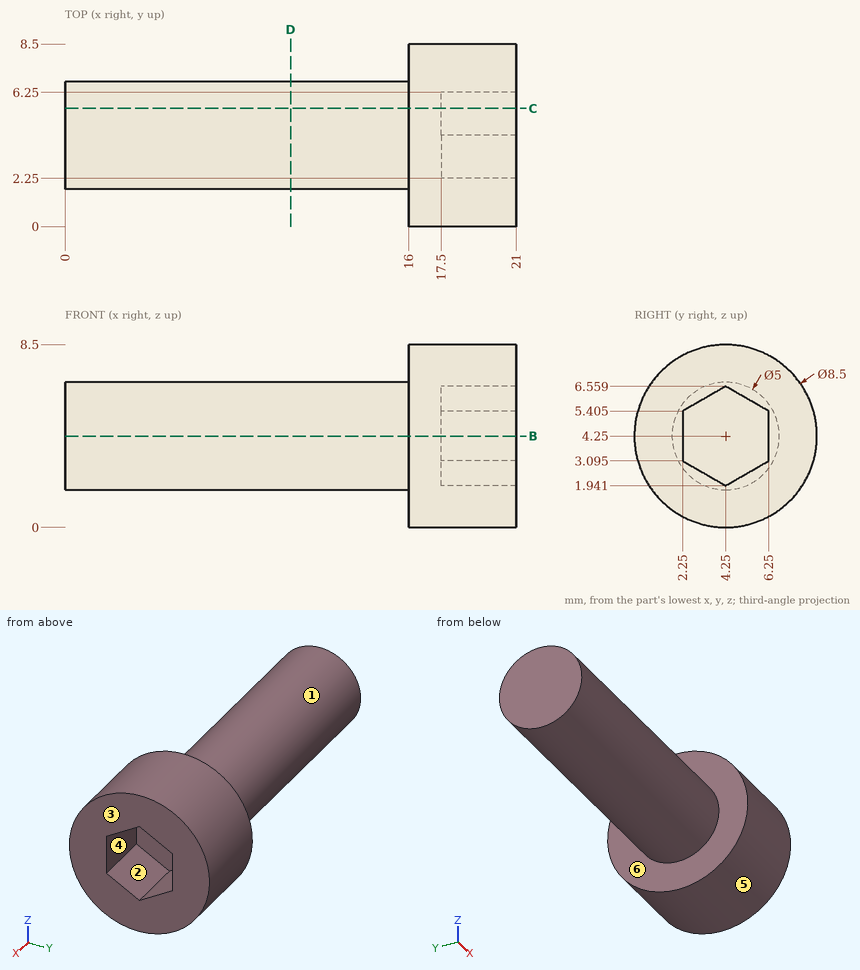
Study the drawing (mm; zero at the part's minimum x, y, z) and answer. A direction names the side the tool comes from. Give positions to 0.01 mm unless a question says otherwise; leave off trailing zeros. Write each loop counter-clockwise with the first axis right and the second up, starting at its lowest first coordinate (ties: lowest second). Pieces come first, ordered by that corner, then holes. Notation, with made-up numbers: (56.25, 73) - (78.25, 73) arc R30 cw to (78.25, 108) - close; hole circle Ø11 at (-4.75, -17). An arc over 180 degrees is marked (long way). Use CSV: the item, a comma, the result in double quotes. Start each with the question number.
(1) Find section C-C (y = 5.5). Give the vertices of the cut face in (x, z) (1 decimal).
(2) Find section D-D (x = 10.5). Give the vertices of the cut face in (y, z).
(3) Given P1, Ø2, axis at x = 11.5, y = 6.5, coming from the -Z side (1 decimal); P2, Ø1, axis at x = 11.5, y = 2, coming from the -Z side (1 decimal); P3, Ø1, axis at x = 7, z = 2.5, coming from the +Y side (1 decimal), each flat-ended and moving along its own axis, determine where each tip first touches the part or whether it passes through.
(4) Determine the mould class of the marked faces 4, 5 and 6 for opening direction Z: +Z half, -Z half, draft (parallel to the pull), parting line (faces both ways), or undercut.
(5) For the marked faces 1, 2 and 3, determine the directions among +Z, -Z, +X, -X, +Y, -Y from which every point of the face is accessible in a straight line to the end or side of a thin tool.
(6) Consider line 1 along X through (y, z) = (3, 1.75); line 2 along Z through (x, y) = (19, 0.5); line 3 along Y through (x, z) = (19.25, 1.25). Determine where each line is inside the solid, lowest interval first.
(7) Find section B-B (z = 4.25). Give the vertices of the cut face in (x, y).
Findings below:
1,outline,"(0, 2.1) - (16, 2.1) - (16, 0.2) - (21, 0.2) - (21, 2.7) - (17.5, 2.7) - (17.5, 5.8) - (21, 5.8) - (21, 8.3) - (16, 8.3) - (16, 6.4) - (0, 6.4) - close"
2,outline,"circle Ø5 at (4.25, 4.25)"
3,P1,"z = 2.1"
3,P2,"z = 2.5"
3,P3,"y = 6.4"
4,face 4,"undercut"
4,face 5,"parting line"
4,face 6,"draft"
5,face 1,"-X"
5,face 2,"+X"
5,face 3,"+Z, -Z, +X, +Y, -Y"
6,line 1,"16 to 21"
6,line 2,"2.25 to 6.25"
6,line 3,"1.24 to 7.26"
7,outline,"(0, 1.75) - (16, 1.75) - (16, 0) - (21, 0) - (21, 2.25) - (17.5, 2.25) - (17.5, 6.25) - (21, 6.25) - (21, 8.5) - (16, 8.5) - (16, 6.75) - (0, 6.75) - close"
